Geometry: see drawing. Coordinates: mm, zero at the bounding-box minimum. Round coordinates to 2 decimals unless told otherwise and drop trailing zeros.
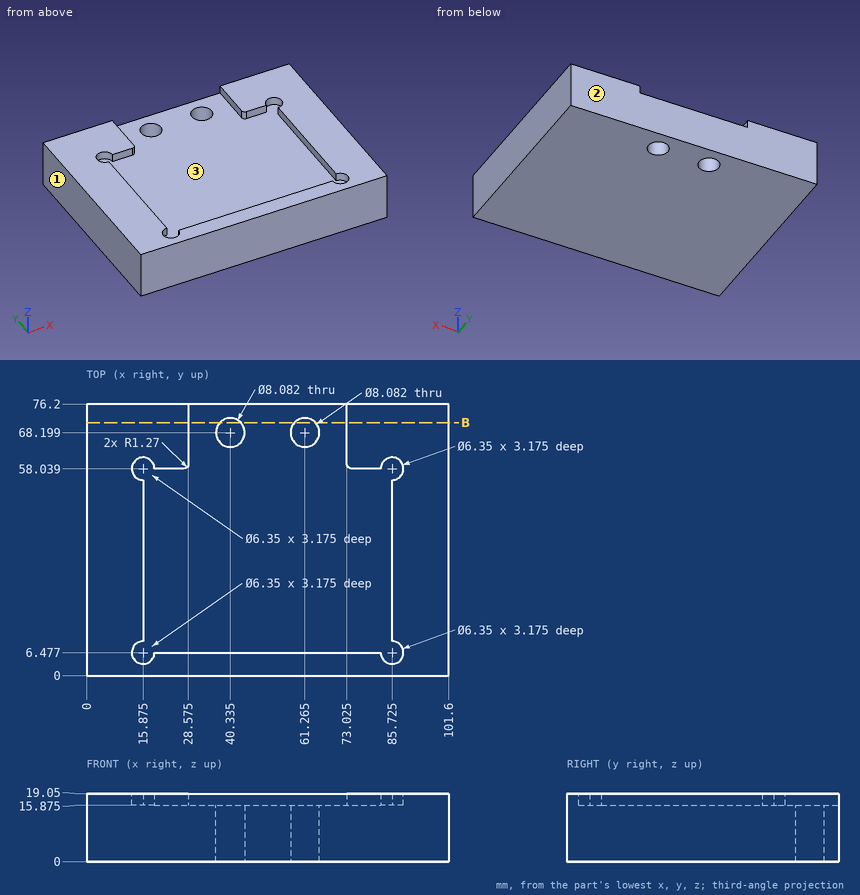
1) Section query B-B on y = 71. State how many separate pieces and enclosed holes the cut face has, then the cut area to 3 significant figures.
Taken from the geometry:
separate pieces: 3
enclosed holes: 0
area: 1,610 mm2
2) Contact query for flat-ended pins moving along their axis: P1, Ø2, axis at x = 46.5, y = 24, coming from the +Z side (3 decimals); P2, Ø1.6, axis at x = 36, z = 18, coming from the +Y side. Output: stop coordinate, or through.
Taken from the geometry:
P1: stops at z = 15.875
P2: stops at y = 6.48
3) Pull-direction query (Y, two-part tool) for the marked faces 1, 2 and 3; classes: released by +Y, released by -Y, zero draft, split by the parting line, or undercut.
Taken from the geometry:
face 1: zero draft
face 2: released by +Y
face 3: undercut
4) Material intervals for line 1 (Z direction, x = 85.5, y = 37) (1 decimal); line 2 (X direction, y = 42.5, z = 16.25) (1 decimal); line 3 (Y direction, x = 51, z = 18.25), sorted ascending.
Taken from the geometry:
line 1: z = 0 to 15.9
line 2: x = 0 to 15.9, 85.7 to 101.6
line 3: y = 0 to 6.48
